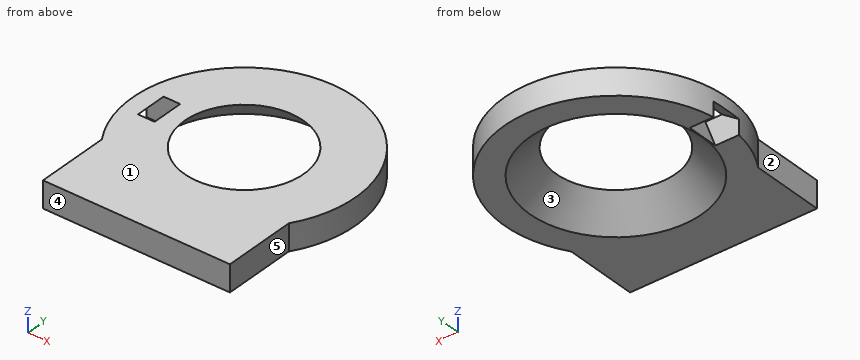
from build123d import *

# Parameters (mm, degrees)
BOSS_EXTRUDE1_DEPTH = 10
SKETCH4_R           = 22.437608593
CUT_EXTRUDE1_DEPTH  = 30
CHAMFER1_SIZE       = 10


with BuildPart() as part:
    # Sketch1 → Boss-Extrude1 (new body)
    with BuildSketch(Plane.XY):
        with BuildLine():
            Line((-35.220966732, -22.879761853), (-35.220966732, -50.5))
            Line((-35.220966732, -50.5), (35.220966732, -50.5))
            Line((35.220966732, -50.5), (35.220966732, -22.879761853))
            ThreePointArc((35.220966732, -22.879761853), (0, 42), (-35.220966732, -22.879761853))
        make_face()
    extrude(amount=BOSS_EXTRUDE1_DEPTH)

    # Sketch3 → Cut-Loft1 section 0
    with BuildSketch(Plane.XY.offset(10)):
        with BuildLine():
            Line((-35.164273033, 6), (-28.90529198, 6))
            Line((-28.90529198, 6), (-28.90529198, -6))
            Line((-28.90529198, -6), (-35.164273033, -6))
            Line((-35.164273033, -6), (-35.164273033, 6))
        make_face()
    # Sketch2 → Cut-Loft1 section 1
    with BuildSketch(Plane(origin=(0, 0, 0), x_dir=(-1, 0, 0), z_dir=(0, 0, -1))):
        with BuildLine():
            Line((32.638910343, 6), (49.791813943, 6))
            Line((49.791813943, 6), (49.791813943, -6))
            Line((49.791813943, -6), (32.638910343, -6))
            Line((32.638910343, -6), (32.638910343, 6))
        make_face()
    loft(mode=Mode.SUBTRACT)

    # Sketch4 → Cut-Extrude1 (cut)
    with BuildSketch(Plane(origin=(0, 0, 0), x_dir=(-1, 0, 0), z_dir=(0, 0, -1))):
        Circle(SKETCH4_R)
    extrude(amount=-CUT_EXTRUDE1_DEPTH, mode=Mode.SUBTRACT)

    # Chamfer1
    chamfer1_edges = [part.edges().sort_by_distance(p)[0] for p in [
        (22.437608593, 0, 0),
    ]]
    chamfer(chamfer1_edges, length=CHAMFER1_SIZE - 0.0001)  # a hair under: the kernel refuses the full size


solid = part.part
Read the model definition and answer for the solid it produces. Units are mm, in the model's axes. Face numbers are marked on the shaded views. A direction names the side the tool comes from. Round coordinates to 2 decimals unless told otherwise and drop trailing zeros.
Q1. Each of these flat-tipped pins is pushed along its axis until it touches: pin 1 (10 mm diameter, centred on x = -19, y = 7, fed in from -Z); pin 2 (1 mm diameter, centred on y = -37, z = 3.5, fed in from +X); pin 3 (1 mm diameter, centred on y = -23, z = 4, fed in from -X). Where does it stop, or does it pass through?
Q2. Determine the mould class of the marked faces 3, 4 and 5 for opening direction Y: released by +Y, released by -Y, zero draft, split by the parting line, or undercut.
Q3. Section B-B on y = 0 is taken. Give the number of separate pieces and of enclosed holes in the cut face, and give its area (3 significant figures).
Q4. Which of the six approach directions +Z, -Z, +X, -X, +Y, -Y give full straight-line access (tool end or side, diameter ignored) to the marked faces 1 and 2?
Q5. Consider probe 1 along Z at (x, y) = (27, 2.5); probe 2 along X at (y, z) = (-1, 6); probe 3 along Y at (x, z) = (-32, 9.25). Determine where each line is inside the solid, lowest interval first.
Output:
1. pin 1: stops at z = 7.19
1. pin 2: stops at x = 35.22
1. pin 3: stops at x = -35.46
2. face 3: undercut
2. face 4: released by -Y
2. face 5: zero draft
3. separate pieces: 3
3. enclosed holes: 0
3. area: 195 mm2
4. face 1: +Z, +X, -X, +Y, -Y
4. face 2: +Z, -Z, -X, -Y
5. probe 1: z = 5.32 to 10
5. probe 2: x = -41.99 to -41.02, -30.4 to -26.42, 26.42 to 41.99
5. probe 3: y = -50.5 to -6, 6 to 27.2
